from build123d import *

# Parameters (mm, degrees)
SKETCH1_R           = 101.6
SKETCH1_R_2         = 23.124366549
BOSS_EXTRUDE1_DEPTH = 38.1
CUT_EXTRUDE1_DEPTH  = 63.5
SKETCH3_R           = 1.5
CUT_EXTRUDE4_DEPTH  = 28.902215931
SKETCH4_R           = 12.7


with BuildPart() as part:
    # Sketch1 → Boss-Extrude1 (new body)
    # profile 1 of 2: a face of its own
    with BuildSketch(Plane(origin=(0, 0, 0), x_dir=(0, 0, -1), z_dir=(1, 0, 0))):
        Circle(SKETCH1_R)
        Circle(SKETCH1_R_2, mode=Mode.SUBTRACT)
    # profile 2 of 2: a face of its own
    with BuildSketch(Plane(origin=(0, 0, 0), x_dir=(0, 0, -1), z_dir=(1, 0, 0))):
        with BuildLine():
            ThreePointArc((21.216434585, 9.197784069), (0, 23.124366549), (-21.216434585, 9.197784069))
            Line((-21.216434585, 9.197784069), (0, 9.197784069))
            Line((0, 9.197784069), (21.216434585, 9.197784069))
        make_face()
    extrude(amount=-BOSS_EXTRUDE1_DEPTH)

    # Sketch2 → Cut-Extrude1 (cut)
    with BuildSketch(Plane(origin=(0, 101.6, 0), x_dir=(1, 0, 0), z_dir=(0, 1, 0))):
        with BuildLine():
            ThreePointArc((-14.05, 0), (-15.514466094, 3.535533906), (-19.05, 5))
            Line((-19.05, 5), (-19.05, -5))
            ThreePointArc((-19.05, -5), (-15.514466094, -3.535533906), (-14.05, 0))
        make_face()
        with BuildLine():
            Line((-19.05, -5), (-19.05, 5))
            ThreePointArc((-19.05, 5), (-24.05, 0), (-19.05, -5))
        make_face()
    extrude(amount=-CUT_EXTRUDE1_DEPTH, mode=Mode.SUBTRACT)

    # Sketch3 → Cut-Extrude4 (cut)
    with BuildSketch(Plane(origin=(0, 38.1, 0), x_dir=(1, 0, 0), z_dir=(0, 1, 0))):
        with Locations(Location((-19.05, 0, 0), (0, 0, 270))):
            Circle(SKETCH3_R)
    extrude(amount=-CUT_EXTRUDE4_DEPTH, mode=Mode.SUBTRACT)

    # Sketch4 → Cut-Revolve1 (revolve, cut)
    with BuildSketch(Plane(origin=(0, 0, 0), x_dir=(1, 0, 0), z_dir=(0, 1, 0)), mode=Mode.PRIVATE) as cut_revolve1_sk:
        with Locations((-19.05, -101.6)):
            Circle(SKETCH4_R)
    revolve(cut_revolve1_sk.sketch.rotate(Axis((-18.38763681, 0, 0), (1, 0, 0)), 180), axis=Axis((-18.38763681, 0, 0), (1, 0, 0)), mode=Mode.SUBTRACT)


solid = part.part
The listing builds one solid part. Answer for the finished solid, in the listing's coordinates (mm). A direction names the side the tool comes from. Coordinates: 2 decimals unless noted, no trailing zeros. Write each loop counter-clockwise with the first axis right and the second up, starting at its lowest first coordinate (ties: lowest second). Pieces come first, ordered by that corner, then holes. Notation, with made-up numbers: (10, 65) - (30, 65) arc R13 ccw to (30, 80) - close; hole circle Ø7 at (36.25, -6). An arc over 180 degrees is marked (long way). Put each result on its own line as item: value.
1. Determine the mould class of faces 4 (the face through (-18.783, -23.115, 0.641)), 5 (the face through (-3.131, -99.184, 22.025)), 6 (the face through (-38.1, 24, 1)) for opening direction Z: pulls with the +Z half, pulls with the -Z half, needs draft (parallel to the pull), parting line crosses it, or undercut.
Answer sheet:
face 4: undercut
face 5: parting line crosses it
face 6: needs draft
2. The part is cut by section A-A on y = 0. Give the vertices of the cut face in (x, z).
Answer sheet:
outline: (-38.1, -101.6) - (-31.75, -101.6) arc R12.7 cw to (-6.35, -101.6) - (0, -101.6) - (0, -23.12) - (-38.1, -23.12) - close; (-38.1, 23.12) - (0, 23.12) - (0, 101.6) - (-6.35, 101.6) arc R12.7 cw to (-31.75, 101.6) - (-38.1, 101.6) - close
3. A tool of negligible diameter and unlimited length cuts with its end or side. For faces 1 (the face through (-23, 9.198, 0)), 2 (the face through (0, 24, 1)), 3 (the face through (-20.2, 38.1, -1.2)), from which of +Z, -Z, +X, -X, +Y, -Y can it reach the whole face along a straight path? Write none if from no direction.
Answer sheet:
face 1: +X, -X
face 2: +Z, -Z, +X, +Y, -Y
face 3: +Y
4. Flat-ended cylindrical pins translate along their axes: pin 1 Ø1.5 at (x, y) = (-7, -20) entering from -Z; pin 2 Ø4 at (x, z) = (-19.05, 0) entering from +Y; pin 3 Ø10 at (x, z) = (-15, -3) entering from -Y. Find the tip coordinate at first contact, or state that the pin passes through.
Answer sheet:
pin 1: stops at z = -99.69
pin 2: stops at y = 38.1
pin 3: stops at y = -92.64
5. Find the intervals of material crossed by line 1 along X through (y, z) = (31.5, 0); line 2 along X through (y, z) = (91.5, -42); line 3 along Y through (x, z) = (-29, 0), in increasing order. Write a range as from..to.
Answer sheet:
line 1: x = -38.1..-20.55, -17.55..0
line 2: x = -38.1..-31.72, -6.38..0
line 3: y = -93.71..-23.12, 9.2..93.71
